```python
from build123d import *

# Parameters (mm, degrees)
F1_DEPTH = 25
F2_R     = 1.5


with BuildPart() as f1:
    # F0 (on Top) → F1 (new body)
    with BuildSketch(Plane.XY):
        with BuildLine():
            Line((0, 32), (0, 1.5))
            Line((0, 1.5), (0, 1.315183))
            ThreePointArc((0, 1.315183), (0.372135, 0.326284), (1.303896, -0.171942))
            Line((1.303896, -0.171942), (35, -4.615385))
            Line((35, -4.615385), (35, 0))
            Line((35, 0), (49, 0))
            Line((49, 0), (49, -6.461538))
            Line((49, -6.461538), (91, -12))
            Line((91, -12), (91, -20.5))
            ThreePointArc((91, -20.5), (91.43934, -21.56066), (92.5, -22))
            Line((92.5, -22), (102, -22))
            ThreePointArc((102, -22), (104.12132, -21.12132), (105, -19))
            Line((105, -19), (105, 0))
            Line((105, 0), (105, 1.5))
            Line((105, 1.5), (105, 51))
            ThreePointArc((105, 51), (104.12132, 53.12132), (102, 54))
            Line((102, 54), (92.5, 54))
            ThreePointArc((92.5, 54), (91.43934, 53.56066), (91, 52.5))
            Line((91, 52.5), (91, 44))
            Line((91, 44), (49, 38.461538))
            Line((49, 38.461538), (49, 32))
            Line((49, 32), (35, 32))
            Line((35, 32), (35, 36.615385))
            Line((35, 36.615385), (0, 32))
        make_face()
    extrude(amount=F1_DEPTH)

    # F2
    f2_edges = [f1.edges().sort_by_distance(p)[0] for p in [
        (0, 32, 12.5),
    ]]
    fillet(f2_edges, radius=F2_R)


solid = f1.part
```
The model under review builds one solid part; all positions refer to its coordinate system, in mm. A direction names the side the tool comes from. Round coordinates to 2 decimals unless told otherwise and drop trailing zeros. Loops run counter-clockwise (first coordinate to the right, second up) from the corner with the lowest first, then second, coordinate; pieces in that order, holes last. Notation, with made-up numbers: (20, 44) -> (57, 44) arc R14 ccw to (57, 49) -> close; hole circle Ø6 at (47.5, 1). An arc over 180 degrees is marked (long way). Answer as a JSON object with one key per item and string values. Group by question number.
1) For pin 1 Ø5 at (x, z) = (18, 5) entering from -Y; pin 2 Ø7 at (y, z) = (35.5, 17.5) entering from -X; pin 3 Ø2.5 at (y, z) = (48, 12.5) entering from -X; pin 4 Ø5 at (x, y) = (76.5, 20) entering from -Z, all flat-tipped, find the tip position at first contact; note any pin that passes through.
2) We need section B-B on y = 48.5. Write out the cut boundary in (x, z), then the cut area to 3 significant figures.
3) Mouldability with a two-part tool opening along X and no side actions: class faces 4 (the face through (91, 48, 12)), 5 (the face through (104.1, -21.14, 12.32)), 6 (the face through (35, -2, 12)) as released by +X, released by -X, zero draft, split by the parting line, or undercut.
4) We need section C-C on x = 43. Write out the cut boundary in (y, z).
5) For faces 1 (the face through (49, 35, 12)), 2 (the face through (91, -16, 12)), 3 (the face through (42, 0, 12)), list the 3-axis set-ups (+Z, -Z, +X, -X, +Y, -Y) from which the entire face can be reached by the end or side of a thin tool; tool diameter is ignored.
6) For line 1 (Y direction, x = 48, z = 17.75); line 2 (Y direction, x = 14, z = 7.25); line 3 (X direction, y = 51.5, z = 20), list the stretches that pass through material, from the lowest coordinate up. Write a range as [from, to].
7) We need section A-A on z = 15.25. Write out the cut boundary in (x, y), then the cut area to 3 significant figures.
Result set:
{
 "1": {"pin 1": "y = -2.7", "pin 2": "x = 0.78", "pin 3": "x = 91", "pin 4": "z = 0"},
 "2": {"outline": "(91, 0) -> (105, 0) -> (105, 25) -> (91, 25) -> close", "area": "350 mm²"},
 "3": {"face 4": "released by -X", "face 5": "released by +X", "face 6": "undercut"},
 "4": {"outline": "(0, 0) -> (32, 0) -> (32, 25) -> (0, 25) -> close"},
 "5": {"face 1": "+Z, -Z, +Y", "face 2": "+Z, -Z, -X, -Y", "face 3": "+Z, -Z, -Y"},
 "6": {"line 1": "[0, 32]", "line 2": "[-1.85, 33.85]", "line 3": "[91, 104.96]"},
 "7": {"outline": "(0, 1.32) arc R1.5 ccw to (1.3, -0.17) -> (35, -4.62) -> (35, 0) -> (49, 0) -> (49, -6.46) -> (91, -12) -> (91, -20.5) arc R1.5 ccw to (92.5, -22) -> (102, -22) arc R3 ccw to (105, -19) -> (105, 51) arc R3 ccw to (102, 54) -> (92.5, 54) arc R1.5 ccw to (91, 52.5) -> (91, 44) -> (49, 38.46) -> (49, 32) -> (35, 32) -> (35, 36.62) -> (1.3, 32.17) arc R1.5 ccw to (0, 30.68) -> close", "area": "4,910 mm²"}
}
